Model file for the job. Use its own axes, mm. Face numbers are marked on the shaded views. Give positions to 0.01 mm unless a question says otherwise; leave off trailing zeros. Order: outer loops, then holes, each group sorted by start corner. A loop starts at its lowest first (then second) coordinate and runs counter-clockwise, first axis right, second up. Notation, with made-up numbers: (82, 42) -> (138, 42) arc R5 ccw to (138, 47) -> close; hole circle Ø4 at (48, 68). An arc over 180 degrees is marked (long way). Use CSV: the item, a comma, the result in double quotes. Start each with the question number.
1. Drop a flat-ended pin along its axis: pin 1 (1.5 mm diameter, centred on x = 1, y = -9, fed in from +Z). Give the stop position or say it passes through.
2. Cut at B-B on x = 0. List the corners of the cut face in (y, z), then the cut area to 3 significant figures.
3. Wall check: line 1 (X direction, y = 17.25, z = 10); line 2 (Z direction, x = 0, y = 15); line 3 (X direction, y = -15, z = 11.75). Give the ranges that are in metal, low to high. Write a range as from..to.
4. Cut at A-A on y = 0. List the corners of the cut face in (x, z), then the cut area to 3 significant figures.
5. Cut at C-C on z = 10. List the corners of the cut face in (x, y).
6. Cut at D-D on z = 17. List the corners of the cut face in (x, y), then the cut area to 3 significant figures.
7. Pull direction Z, two halves, no side cores. Call the marked faces 1, 2, 3 and 4: released by +Z, released by -Z, zero draft, split by the parting line, or undercut.
```python
from build123d import *

# Parameters (mm, degrees)
IZIM1_W                     = 30
IZIM1_H                     = 50
IZIM1_R                     = 10
Y_KSEKLIK_EKSTR_ZYON1_DEPTH = 20
KES_EKSTR_ZYON1_REACH       = 57.902
IZIM2_R                     = 2.5


with BuildPart() as part:
    # Çizim1 → Yükseklik-Ekstrüzyon1 (new body)
    with BuildSketch(Plane.XY):
        Rectangle(IZIM1_W, IZIM1_H)
        Circle(IZIM1_R, mode=Mode.SUBTRACT)
    extrude(amount=Y_KSEKLIK_EKSTR_ZYON1_DEPTH)

    # Kes-Ekstrüzyon1: up to this face of the body (flat: up to its plane)
    kes_ekstr_zyon1_end = Plane(part.part.faces().sort_by_distance((0, -25, 10))[0])
    # Çizim2 → Kes-Ekstrüzyon1 (cut, up to the picked face)
    with BuildSketch(Plane(origin=(0, 25, 0), x_dir=(1, 0, 0), z_dir=(0, 1, 0)), mode=Mode.PRIVATE) as kes_ekstr_zyon1_sk1:
        with Locations(Location((0, -10, 0), (0, 0, 180))):
            Circle(IZIM2_R)
    kes_ekstr_zyon1_tool1 = split(extrude(kes_ekstr_zyon1_sk1.sketch, amount=-KES_EKSTR_ZYON1_REACH, mode=Mode.PRIVATE), bisect_by=kes_ekstr_zyon1_end, keep=Keep.BOTH, mode=Mode.PRIVATE)
    add(kes_ekstr_zyon1_tool1.solids().sort_by(Axis((0, 25, 10), (0, -1, 0)))[0], mode=Mode.SUBTRACT)


solid = part.part
```
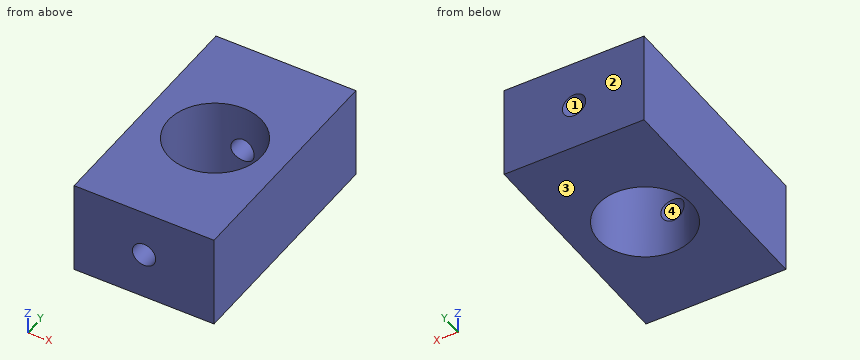
Verdict:
1,pin 1,"through"
2,outline,"(-25, 0) -> (-10, 0) -> (-10, 7.5) -> (-25, 7.5) -> close; (-25, 12.5) -> (-10, 12.5) -> (-10, 20) -> (-25, 20) -> close; (10, 0) -> (25, 0) -> (25, 7.5) -> (10, 7.5) -> close; (10, 12.5) -> (25, 12.5) -> (25, 20) -> (10, 20) -> close"
2,area,"450 mm^2"
3,line 1,"-15..-2.5, 2.5..15"
3,line 2,"0..7.5, 12.5..20"
3,line 3,"-15..-1.79, 1.79..15"
4,outline,"(-15, 0) -> (-10, 0) -> (-10, 20) -> (-15, 20) -> close; (10, 0) -> (15, 0) -> (15, 20) -> (10, 20) -> close"
4,area,"200 mm^2"
5,outline,"(-15, -25) -> (-2.5, -25) -> (-2.5, -9.68) arc R10 cw to (-2.5, 9.68) -> (-2.5, 25) -> (-15, 25) -> close; (2.5, -25) -> (15, -25) -> (15, 25) -> (2.5, 25) -> (2.5, 9.68) arc R10 cw to (2.5, -9.68) -> close"
6,outline,"(-15, -25) -> (15, -25) -> (15, 25) -> (-15, 25) -> close; hole circle Ø20 at (0, 0)"
6,area,"1,190 mm^2"
7,face 1,"undercut"
7,face 2,"zero draft"
7,face 3,"released by -Z"
7,face 4,"undercut"
